Build history of the part. All positions in model axes, mm. A direction names the side the tool comes from. Round coordinates to 2 decimals unless told otherwise and drop trailing zeros. Write each loop counter-clockwise with the first axis right and the second up, starting at its lowest first coordinate (ties: lowest second). Pieces come first, ordered by that corner, then holes. Notation, with made-up numbers: M -17,-22.5 L 31,-22.5 A23 cw 31,-0.5 Z; hole C 36.5,-4.5 d8. An arc over 180 degrees is marked long. Write item = value, one per line. Start each with the question number.
Q1. Pull direction X, two halves, no side cores. Call faces 3 (the flat face through (20, 0, 210)), 4 (the flat face through (19.7, -0.2, 0)), 5 (the flat face through (-3, 2, 210)): released by +X, released by -X, zero draft, split by the parting line, or undercut.
Q2. Tool access for faces 1 (the flat face through (0, 3, 210)), 2 (the flat face through (19.7, -0.2, 425)): list every direction of +Z, -Z, +X, -X, +Y, -Y with a clear straight run to the whole face (end or side of a thin tool).
Q3. Band-saw the part on C-C on x = 4. Write the cut outline in (y, z).
Q4. Band-saw the part on A-A on y = 3.5. Write the cut outline in (x, z), plus the area to 3 significant figures.
Q5. Band-saw the part on B-B on z = 140. Write the cut outline in (x, y).
Q6. Probe L1, parallel to X at y = -0.7, z = 361.5; L2, parallel to X at y = 2.5, z = 286; L3, parallel to Z at x = 10, y = -1.2. List the from-to ranges inside material, lowest first.
```python
from build123d import *

# Parameters (mm, degrees)
BOSS_EXTRUDE1_DEPTH       = 425
F_3_0MM_DOWEL_HOLE1_D     = 3
F_3_0MM_DOWEL_HOLE1_DEPTH = 15
F_3_0MM_DOWEL_HOLE1_TIP   = 0.901290929
F_3_0MM_DOWEL_HOLE2_D     = 3
F_3_0MM_DOWEL_HOLE2_DEPTH = 15
F_3_0MM_DOWEL_HOLE2_TIP   = 0.901290929


with BuildPart() as part:
    # Sketch1 → Boss-Extrude1 (new body)
    with BuildSketch(Plane.XY):
        Polygon((0, 0), (0, 7), (-3, 7), (-3, -3), (43, -3), (43, 7), (40, 7), (40, 0), align=None)
    extrude(amount=BOSS_EXTRUDE1_DEPTH)

    # Ø3.0mm Dowel Hole1
    with Locations(Plane(origin=(0, 0, 0), x_dir=(1, 0, 0), z_dir=(0, 1, 0))):
        with Locations((10, -375.5), (30, -375.5), (30, -361.5), (10, -361.5)):
            Hole(F_3_0MM_DOWEL_HOLE1_D / 2, depth=F_3_0MM_DOWEL_HOLE1_DEPTH)
            with Locations((0, 0, -(F_3_0MM_DOWEL_HOLE1_DEPTH + F_3_0MM_DOWEL_HOLE1_TIP / 2))):  # 118° drill point
                Cone(0, F_3_0MM_DOWEL_HOLE1_D / 2, F_3_0MM_DOWEL_HOLE1_TIP, mode=Mode.SUBTRACT)

    # Ø3.0mm Dowel Hole2
    with Locations(Plane(origin=(0, -3, 0), x_dir=(-1, 0, 0), z_dir=(0, -1, 0))):
        with Locations((-30, -417), (-10, -417)):
            Hole(F_3_0MM_DOWEL_HOLE2_D / 2, depth=F_3_0MM_DOWEL_HOLE2_DEPTH)
            with Locations((0, 0, -(F_3_0MM_DOWEL_HOLE2_DEPTH + F_3_0MM_DOWEL_HOLE2_TIP / 2))):  # 118° drill point
                Cone(0, F_3_0MM_DOWEL_HOLE2_D / 2, F_3_0MM_DOWEL_HOLE2_TIP, mode=Mode.SUBTRACT)


solid = part.part
```
Conclusion:
q1.face_3 = undercut
q1.face_4 = zero draft
q1.face_5 = released by -X
q2.face_1 = +Z, -Z, +Y
q2.face_2 = +Z, +X, -X, +Y, -Y
q3.outline = M -3,0 L 0,0 L 0,425 L -3,425 Z
q4.outline = M -3,0 L 0,0 L 0,425 L -3,425 Z; M 40,0 L 43,0 L 43,425 L 40,425 Z
q4.area = 2,550 mm^2
q5.outline = M -3,-3 L 43,-3 L 43,7 L 40,7 L 40,0 L 0,0 L 0,7 L -3,7 Z
q6.L1 = -3 to 8.5, 11.5 to 28.5, 31.5 to 43
q6.L2 = -3 to 0, 40 to 43
q6.L3 = 0 to 360, 363 to 374, 377 to 415.5, 418.5 to 425
